Read the model definition and answer for the solid it produces. Units are mm, in the model's axes. A direction names the side the tool comes from. Coordinates: 2 decimals unless noted, no trailing zeros. Loops run counter-clockwise (first coordinate to the right, second up) from the corner with the lowest first, then second, coordinate; pieces in that order, holes last.
Autodesk Inventor part; units mm, degrees
ref_plane "Work Plane1" through (59.5, 40.5, 19) normal (-0.7071, -0.7071, 0) x (-0.7071, 0.7071, 0)
ref_plane "YZ Plane" through (0, 0, 0) normal (1, 0, 0) x (0, 1, 0)
ref_plane "XZ Plane" through (0, 0, 0) normal (0, 1, 0) x (-1, 0, 0)
sketch "Sketch1" plane through (0, 0, 0) normal (0, 0, 1) x (1, 0, 0)
  line L0 (0, 0) -> (100, 0) construction
  line L1 (100, 0) -> (100, 100) construction
  line L2 (100, 100) -> (0, 100) construction
  line L3 (0, 100) -> (0, 0) construction
  line L4 (0, 0) -> (100, 100)
  line L5 (0, 0) -> (19, 0)
  line L6 (100, 100) -> (100, 81)
  line L7 (19, 0) -> (100, 81)
  dimension "d1" = 100
  dimension "d2" = 100
  dimension "d3" = 19
  dimension "d4" = 19
extrude "Extrusion1" add sketch "Sketch1" along normal blind 19
ref_plane "Work Plane1" through (59.5, 40.5, 19) normal (-0.7071, -0.7071, 0) x (-0.7071, 0.7071, 0)
sketch "Sketch2" plane through (59.5, 40.5, 19) normal (-0.7071, -0.7071, 0) x (-0.7071, 0.7071, 0)
  line L0 (13.435, 19) -> (0, 19)
  line L1 (13.435, 19) -> (13.435, 0)
  line L2 (0, 0) -> (13.435, 0)
  line L3 (0, 19) -> (0, 0)
  line L4 (11.935, 1.5) -> (11.935, 17.5)
  line L5 (11.935, 17.5) -> (1.5, 17.5)
  line L6 (1.5, 17.5) -> (1.5, 1.5)
  line L7 (1.5, 1.5) -> (11.935, 1.5)
  point P0 (13.435, 19)
  dimension "d7" = 1.5
extrude "Extrusion2" cut sketch "Sketch2" along normal through all both and the other way through all contours L7 L6 L5 L4
sketch "Sketch4" plane through (0, 0, 19) normal (0, 0, 1) x (1, 0, 0)
  line L0 (36.3882, 26.4887) -> (73.5113, 63.6118) construction
  line L1 (54.9497, 45.0503) -> (50, 50) construction
  line L2 (100, 100) -> (0, 0) construction
  circle A0 centre (36.3882, 26.4887) radius 1.5
  circle A1 centre (73.5113, 63.6118) radius 1.5
  line L3 (19, 0) -> (100, 81)
  dimension "d22" = 52.5
  dimension "d24" = 7
  dimension "d25" = 3
  dimension "d26" = 3
extrude "Extrusion4" cut sketch "Sketch4" against normal through all
sketch "Sketch5" plane through (100, 81, 19) normal (0.7071, -0.7071, 0) x (-0.7071, -0.7071, 0)
  line L0 (92.2756, 9) -> (22.2756, 9) construction
  line L1 (0, 19) -> (114.5513, 19)
  circle A0 centre (92.2756, 9) radius 1.5
  circle A1 centre (22.2756, 9) radius 1.5
  point P0 (127.9863, 19)
  point P1 (57.2756, 19)
  point P2 (57.2756, 9)
  dimension "d29" = 70
  dimension "d30" = 10
  dimension "d31" = 3
  dimension "d32" = 3
extrude "Extrusion5" cut sketch "Sketch5" against normal through all
properties part number "C002" material "Aluminum 6061"
Q1. A cutting plane is placed at B-B (y = 33). Give the vertices of the cut face in (x, z), then the cut area to 3 significant figures.
Findings below:
outline: (33, 0) - (52, 0) - (52, 19) - (33, 19) - close; hole (35.12, 1.5) - (49.88, 1.5) - (49.88, 17.5) - (35.12, 17.5) - close
area: 125 mm2
Q2. Flat-ended cylindrical pins translate along their axes: pin 1 Ø10 at (y, z) = (31, 7.5) entering from -X; pin 2 Ø10 at (y, z) = (35.5, 9) entering from -X; pin 3 Ø4 at (x, y) = (36.39, 26.49) entering from -Z; pin 4 Ø10 at (y, z) = (78, 15.5) entering from -X. Find the tip coordinate at first contact, or state that the pin passes through.
Findings below:
pin 1: stops at x = 26
pin 2: stops at x = 30.5
pin 3: stops at z = 0
pin 4: stops at x = 73
Q3. Determine the mould class of faces 1 (the face through (53, 43, 19)), 2 (the face through (72.32, 62.7, 0.76)), 3 (the face through (55, 46, 17.5)) for opening direction Z: +Z half, -Z half, draft (parallel to the pull), parting line (faces both ways), or undercut.
Findings below:
face 1: +Z half
face 2: draft
face 3: undercut
Q4. Which of the six approach directions +Z, -Z, +X, -X, +Y, -Y give full straight-line access (tool end or side, diameter ignored) to faces 4 (the face through (55, 46, 1.5)), 5 (the face through (100, 82, 9))?
Findings below:
face 4: none
face 5: +Z, -Z, +X, +Y, -Y
Q5. A cutting plane is placed at A-A (z = 13). Give the vertices of the cut face in (x, y).
Findings below:
outline: (0, 0) - (2.12, 0) - (100, 97.88) - (100, 100) - close; (16.88, 0) - (19, 0) - (100, 81) - (100, 83.12) - close
Q6. A cutting plane is placed at D-D (x = 65.5). Give the vertices of the cut face in (y, z).
Findings below:
outline: (46.5, 0) - (65.5, 0) - (65.5, 19) - (46.5, 19) - close; hole (48.62, 1.5) - (63.38, 1.5) - (63.38, 17.5) - (48.62, 17.5) - close
Q7. Straight lines are drawn through the part: probe 1 along Z at (x, y) = (26.5, 21); probe 2 along Y at (x, z) = (95, 5.75); probe 3 along Y at (x, z) = (81, 3.5). For each, find the intervals that lie inside material, in ascending order.
Findings below:
probe 1: z = 0 to 1.5, 17.5 to 19
probe 2: y = 76 to 78.12, 92.88 to 95
probe 3: y = 62 to 64.12, 78.88 to 81
Q8. A cutting plane is placed at C-C (x = 15.5). Give the vertices of the cut face in (y, z).
Findings below:
outline: (0, 0) - (15.5, 0) - (15.5, 19) - (0, 19) - (0, 17.5) - (13.38, 17.5) - (13.38, 1.5) - (0, 1.5) - close
